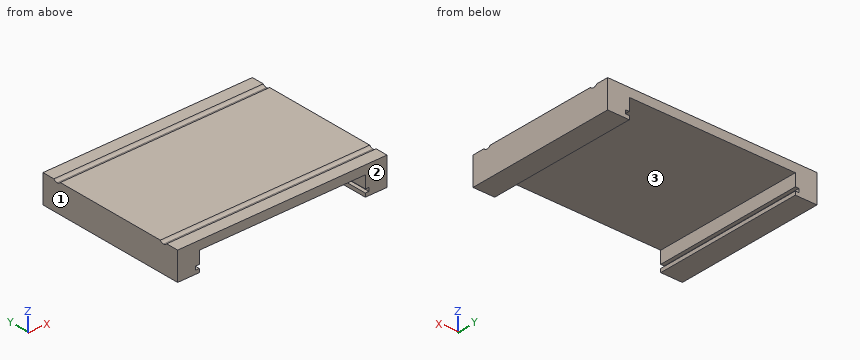
from build123d import *

# Parameters (mm, degrees)
F0_W     = 290
F0_H     = 210
F1_DEPTH = 12
F2_W     = 30
F2_H     = 210
F3_DEPTH = 27
F4_W     = 5
F4_H     = 5
F5_DEPTH = 210.001
F7_DEPTH = 290.001


# Not quite as in the source:
# - a pattern or mirror of a feature is missing from the dataset's text; its kind, count and spacing are read off the source's solid


with BuildPart() as f1:
    # F0 (on Top) → F1 (new body)
    with BuildSketch(Plane.XY):
        Rectangle(F0_W, F0_H)
    extrude(amount=-F1_DEPTH)

    # F2 (on face) → F3 (join)
    with BuildSketch(Plane(origin=(0, 0, -12), x_dir=(1, 0, 0), z_dir=(0, 0, -1))):
        with Locations((130, 0)):
            Rectangle(F2_W, F2_H)
        with Locations((-130, 0)):
            Rectangle(F2_W, F2_H)
    extrude(amount=F3_DEPTH)

    # F4 (on face) → F5 (cut, through all)
    with BuildSketch(Plane.XZ.offset(105)):
        with Locations((-117.5, -31.5)):
            Rectangle(F4_W, F4_H)
        with Locations((117.5, -31.5)):
            Rectangle(F4_W, F4_H)
    extrude(amount=-F5_DEPTH, mode=Mode.SUBTRACT)

    # F6 (on face) → F7 (cut, through all)
    with BuildSketch(Plane(origin=(-145, 0, 0), x_dir=(0, -1, 0), z_dir=(-1, 0, 0))):
        with BuildLine():
            Line((-78, 0), (-88, 0))
            ThreePointArc((-88, 0), (-85.7950849719, -1.8401699437), (-83, -2.5))
            ThreePointArc((-83, -2.5), (-80.2049150281, -1.8401699437), (-78, 0))
        make_face()
    f7 = extrude(amount=-F7_DEPTH, mode=Mode.SUBTRACT)

    # F7_copies: F7 across plane
    add(f7.mirror(Plane(origin=(0, 0, 0), x_dir=(0, 0, -1), z_dir=(0, -1, 0))), mode=Mode.SUBTRACT)


solid = f1.part
Geometry check sheet. Reference: the model listing, model coordinates, mm. Face numbers are marked on the shaded views. Give positions to 0.01 mm unless a question says otherwise; leave off trailing zeros. Write each loop counter-clockwise with the first axis right and the second up, starting at its lowest first coordinate (ties: lowest second). Pieces come first, ordered by that corner, then holes. Notation, with made-up numbers: M 21,14 L 62,14 A27 cw 62,45 Z; hole C 25.25,75.5 d6. An arc over 180 degrees is marked long. Answer as CSV lines item,"result". Start each with the question number.
Q1. Material ranges on L1, parallel to X at y = -47, z = -22; L2, parallel to X at y = -74, z = -33.5; L3, parallel to Z at x = 67.5, y = 55.5, recorded low to high.
Q2. Section check B-B, the plane y = 26.5. Record the cut outline in (x, z), then the cut area to 3 significant figures.
Q3. Release check for a two-part mould opening along X. For the marked faces 1, 2 and 3 record: pulls with the +X half, pulls with the -X half, needs draft (parallel to the pull), parting line crosses it, or undercut.
Q4. Go/stop test with flat-tipped pins: pin 1 (1.5 mm diameter, centred on x = -24, y = -69.5, fed in from -Z); pin 2 (12 mm diameter, centred on x = -101.5, z = -17.5, fed in from -Y). Record where each tip stops, or that it passes through.
Q5. Section check C-C, the plane x = 42.5. Record the cut outline in (y, z), then the cut area to 3 significant figures.
Q6. Section check A-A, the plane z = -16.5. Record the cut outline in (x, y), then the cut area to 3 significant figures.
Geometry says:
1,L1,"-145 to -115, 115 to 145"
1,L2,"-145 to -120, 120 to 145"
1,L3,"-12 to 0"
2,outline,"M -145,-39 L -115,-39 L -115,-34 L -120,-34 L -120,-29 L -115,-29 L -115,-12 L 115,-12 L 115,-29 L 120,-29 L 120,-34 L 115,-34 L 115,-39 L 145,-39 L 145,0 L -145,0 Z"
2,area,"5,050 mm^2"
3,face 1,"pulls with the -X half"
3,face 2,"needs draft"
3,face 3,"undercut"
4,pin 1,"z = -12"
4,pin 2,"y = -105"
5,outline,"M -105,-12 L 105,-12 L 105,0 L 88,0 A6.25 cw 78,0 L -78,0 A6.25 cw -88,0 L -105,0 Z"
5,area,"2,490 mm^2"
6,outline,"M -145,-105 L -115,-105 L -115,105 L -145,105 Z; M 115,-105 L 145,-105 L 145,105 L 115,105 Z"
6,area,"12,600 mm^2"
